Read the model definition and answer for the solid it produces. Units are mm, in the model's axes. Face numbers are marked on the shaded views. Coordinates: 2 decimals unless noted, no trailing zeros. Loops run counter-clockwise (first coordinate to the right, second up) from the corner with the lowest first, then second, coordinate; pieces in that order, holes last. Notation, with made-up numbers: (78, 6) - (101, 6) arc R18 cw to (101, 31) - close; hole circle Ø5 at (77.25, -38). An arc over 180 degrees is marked (long way). Use one line per item in the form item = value. Start each with the question number.
1) A cutting plane is placed at A-A (z = 11). Give the vertices of the cut face in (x, y), and give its area (3 significant figures).
2) Consider line 1 (X direction, y = 4.9, z = 44); line 2 (X direction, y = 1.1, z = 44); line 3 (Z direction, x = -39, y = 3.9). Determine where each line is inside the solid, lowest interval first.
3) A cutting plane is placed at B-B (x = 6). Give the vertices of the cut face in (y, z).
4) Each of these flat-tipped pins is pushed along its axis until it touches: P1, Ø0.6, axis at y = -1, z = 1, coming from the +X side; P2, Ø1, axis at x = -15, y = -1, coming from the +Z side; P3, Ø4, axis at x = 39, z = -44, coming from the -Y side. Where does it stop, or does it pass through?
5) The mould has two halves that part along X. Classify the marked faces 1 and 2: released by +X, released by -X, zero draft, split by the parting line, or undercut.
from build123d import *

# Parameters (mm, degrees)
SKETCH1_W           = 90
SKETCH1_H           = 100
BOSS_EXTRUDE1_DEPTH = 3
SKETCH2_R           = 1.7
CUT_EXTRUDE1_DEPTH  = 4
SKETCH4_W           = 80.2
SKETCH4_H           = 93.2
SKETCH4_W_2         = 74.2
SKETCH4_H_2         = 87.2
BOSS_EXTRUDE2_DEPTH = 2
CUT_EXTRUDE5_START  = -3
SKETCH6_R           = 6
CUT_EXTRUDE5_DEPTH  = 3
SKETCH7_W           = 90
SKETCH7_H           = 3
BOSS_EXTRUDE3_DEPTH = 4
SKETCH8_R           = 3.75
BOSS_EXTRUDE4_DEPTH = 2.7
FILLET1_R           = 8


with BuildPart() as part:
    # Sketch1 → Boss-Extrude1 (new body)
    with BuildSketch(Plane(origin=(0, 0, 0), x_dir=(1, 0, 0), z_dir=(0, 1, 0))):
        Rectangle(SKETCH1_W, SKETCH1_H)
    extrude(amount=BOSS_EXTRUDE1_DEPTH)

    # Sketch2 → Cut-Extrude1 (cut, through all)
    with BuildSketch(Plane(origin=(0, 3, 0), x_dir=(1, 0, 0), z_dir=(0, 1, 0))):
        with Locations((-39, 44)):
            Circle(SKETCH2_R)
        with Locations((39, 44)):
            Circle(SKETCH2_R)
        with Locations((39, -44)):
            Circle(SKETCH2_R)
        with Locations((-39, -44)):
            Circle(SKETCH2_R)
    extrude(amount=-CUT_EXTRUDE1_DEPTH, mode=Mode.SUBTRACT)

    # Sketch4 → Boss-Extrude2 (add)
    with BuildSketch(Plane.XZ):
        with Locations((1.5, 0)):
            Rectangle(SKETCH4_W, SKETCH4_H)
        with Locations((1.5, 0)):
            Rectangle(SKETCH4_W_2, SKETCH4_H_2, mode=Mode.SUBTRACT)
    extrude(amount=BOSS_EXTRUDE2_DEPTH)

    # Sketch6 → Cut-Extrude5 (cut, through all)
    with BuildSketch(Plane(origin=(0, 3, 0), x_dir=(1, 0, 0), z_dir=(0, 1, 0)).offset(CUT_EXTRUDE5_START)):
        with Locations((-39, 44)):
            Circle(SKETCH6_R)
        with Locations((-39, -44)):
            Circle(SKETCH6_R)
        with Locations((39, -44)):
            Circle(SKETCH6_R)
        with Locations((39, 44)):
            Circle(SKETCH6_R)
    extrude(amount=-CUT_EXTRUDE5_DEPTH, mode=Mode.SUBTRACT)

    # Sketch7 → Boss-Extrude3 (add)
    with BuildSketch(Plane.XY.offset(50)):
        with Locations((0, 1.5)):
            Rectangle(SKETCH7_W, SKETCH7_H)
    extrude(amount=BOSS_EXTRUDE3_DEPTH)

    # Sketch8 → Boss-Extrude4 (add)
    with BuildSketch(Plane(origin=(0, 3, 0), x_dir=(1, 0, 0), z_dir=(0, 1, 0))):
        Polygon((-45, -50), (-45, -54), (45, -54), (45, -50), (45, 50), (-45, 50), align=None)
        with Locations((-39, 44)):
            Circle(SKETCH8_R, mode=Mode.SUBTRACT)
        with Locations((39, 44)):
            Circle(SKETCH8_R, mode=Mode.SUBTRACT)
        with Locations((-39, -44)):
            Circle(SKETCH8_R, mode=Mode.SUBTRACT)
        with Locations((39, -44)):
            Circle(SKETCH8_R, mode=Mode.SUBTRACT)
    extrude(amount=BOSS_EXTRUDE4_DEPTH)

    # Fillet1
    fillet1_edges = [part.edges().sort_by_distance(p)[0] for p in [
        (-45, 2.85, 54),
        (45, 2.85, 54),
        (-45, 2.85, -50),
        (45, 2.85, -50),
    ]]
    fillet(fillet1_edges, radius=FILLET1_R)


solid = part.part
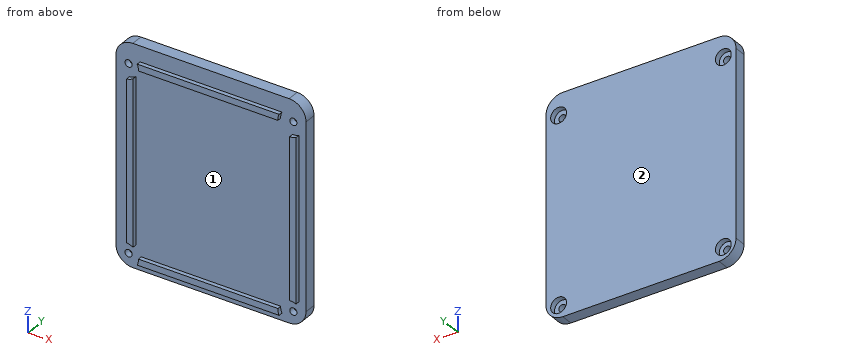
Found:
q1.outline = (-45, 0) - (-38.6, 0) - (-38.6, -2) - (-35.6, -2) - (-35.6, 0) - (38.6, 0) - (38.6, -2) - (41.6, -2) - (41.6, 0) - (45, 0) - (45, 5.7) - (-45, 5.7) - close
q1.area = 525 mm^2
q2.line_1 = -45 to -42.75, -35.25 to 35.25, 42.75 to 45
q2.line_2 = -45 to -40.7, -37.3 to 37.3, 40.7 to 45
q2.line_3 = -49.75 to -47.75, -40.25 to 40.25, 47.75 to 53.75
q3.outline = (-2, -46.6) - (0, -46.6) - (0, -50) - (5.7, -50) - (5.7, 54) - (0, 54) - (0, 46.6) - (-2, 46.6) - (-2, 43.6) - (0, 43.6) - (0, -43.6) - (-2, -43.6) - close
q4.P1 = 41.6
q4.P2 = 46.6
q4.P3 = 0
q5.face_1 = undercut
q5.face_2 = zero draft
